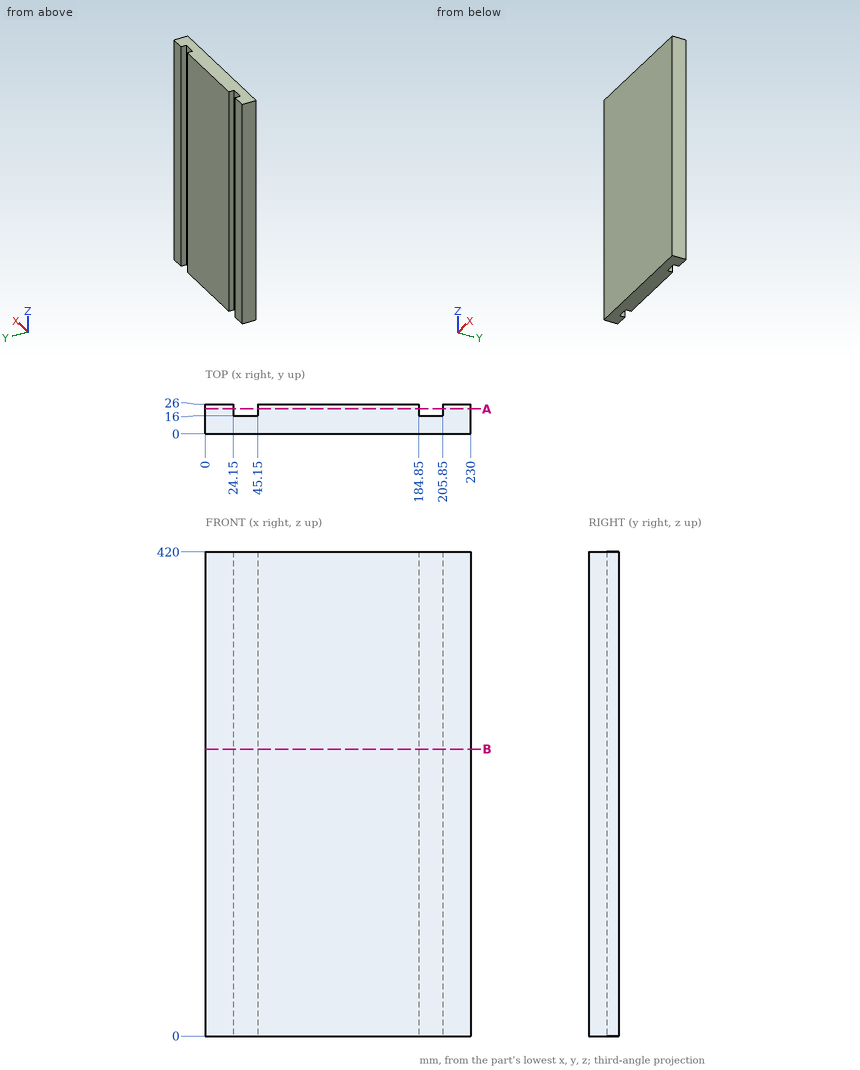
Study the drawing (mm; zero at the part's minimum x, y, z) and answer. Give positions to 0.01 mm unless a question says otherwise; leave off trailing zeros. Loops run counter-clockwise (first coordinate to the right, second up) from the corner with the lowest first, then second, coordinate; pieces in that order, holes last. Notation, with made-up numbers: (70.5, 67.25) - (81.5, 67.25) arc R27 cw to (81.5, 98.25) - close; hole circle Ø1 at (-24.5, 51.25). An arc over 180 degrees is marked (long way). One line per question, with ' | ' between items.
(1) Each of these flat-tipped pins is pushed along its axis until it touches: pin 1 Ø17 at (x, z) = (35, 203.5) entering from +Y; pin 2 Ø11 at (y, z) = (22.5, 296) entering from -X. Where does it stop, or does it pass through?
Recorded:
pin 1: stops at y = 16 | pin 2: stops at x = 0
(2) Straight lines are drawn through the part: probe 1 along X at (y, z) = (18.5, 252); probe 2 along Y at (x, z) = (29, 185). For each, find the intervals that lie inside material, in ascending order.
Recorded:
probe 1: x = 0 to 24.15, 45.15 to 184.85, 205.85 to 230 | probe 2: y = 0 to 16
(3) The part is cut by section A-A (y = 21.75). Write down the section's boundary in (x, z).
Recorded:
outline: (0, 0) - (24.15, 0) - (24.15, 420) - (0, 420) - close; (45.15, 0) - (184.85, 0) - (184.85, 420) - (45.15, 420) - close; (205.85, 0) - (230, 0) - (230, 420) - (205.85, 420) - close
(4) The part is cut by section B-B (z = 249). Write down the section's boundary in (x, y).
Recorded:
outline: (0, 0) - (230, 0) - (230, 26) - (205.85, 26) - (205.85, 16) - (184.85, 16) - (184.85, 26) - (45.15, 26) - (45.15, 16) - (24.15, 16) - (24.15, 26) - (0, 26) - close
